Answer from the drawing. Dimensions are ordinates in mm from the lowest x, y and z of the part. A direction names the side the tool comes from. Round coordinates to 2 decimals unless told otherwise and drop trailing zeros. Order: outer loops, then holes, each group sorted by start corner. A loop starts at its lowest first (then second) coordinate and runs counter-clockwise, first axis right, second up.
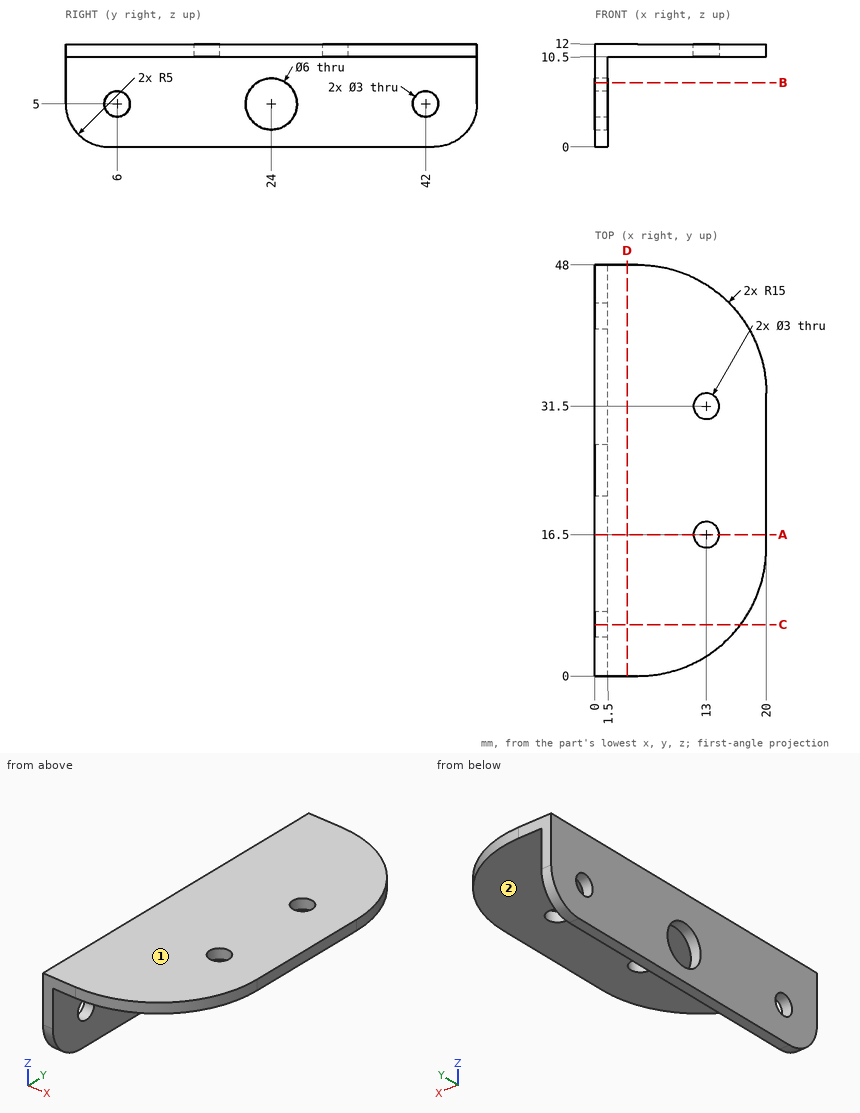
Q1. A cutting plane is placed at D-D, the plane x = 3.75. Give the vertices of the cut face in (y, z), plus the area to 3 significant figures.
Outcome:
outline: (0, 10.5) - (48, 10.5) - (48, 12) - (0, 12) - close
area: 72.0 mm2
Q2. Flat-ended cylindrical pins translate along their axes: pin 1 (4 mm diameter, centred on x = 2.5, z = 7.5, fed in from -Y); pin 2 (3 mm diameter, centred on y = 38.5, z = 8, fed in from +X); pin 3 (5.5 mm diameter, centred on x = 11.5, y = 15, fed in from -Z). Find the tip coordinate at first contact, or state that the pin passes through.
Outcome:
pin 1: stops at y = 0
pin 2: stops at x = 1.5
pin 3: stops at z = 10.5
Q3. For the marked faces 1 and 2, determine the directions among +Z, -Z, +X, -X, +Y, -Y from which every point of the face is accessible in a straight line to the end or side of a thin tool.
Outcome:
face 1: +Z, +X, -X, +Y, -Y
face 2: -Z, +X, +Y, -Y
Q4. Straight lines are drawn through the part: probe 1 along Y at (x, z) = (0.65, 5); probe 2 along Y at (x, z) = (13, 10.95); probe 3 along Z at (x, y) = (0.4, 42). For each, find the intervals that lie inside material, in ascending order.
Outcome:
probe 1: y = 0 to 4.5, 7.5 to 21, 27 to 40.5, 43.5 to 48
probe 2: y = 2.31 to 15, 18 to 30, 33 to 45.69
probe 3: z = 0 to 3.5, 6.5 to 12
Q5. A cutting plane is placed at B-B, the plane z = 7.5. Give the vertices of the cut face in (x, y).
Outcome:
outline: (0, 0) - (1.5, 0) - (1.5, 22.34) - (0, 22.34) - close; (0, 25.66) - (1.5, 25.66) - (1.5, 48) - (0, 48) - close
Q6. A cutting plane is placed at C-C, the plane y = 6. Give the vertices of the cut face in (x, z), plus the area to 4 significant figures.
Outcome:
outline: (0, 0) - (1.5, 0) - (1.5, 3.5) - (0, 3.5) - close; (0, 6.5) - (1.5, 6.5) - (1.5, 10.5) - (17, 10.5) - (17, 12) - (0, 12) - close
area: 36.75 mm2
Q7. A cutting plane is placed at A-A, the plane y = 16.5. Give the vertices of the cut face in (x, z), plus the area to 4 significant figures.
Outcome:
outline: (0, 0) - (1.5, 0) - (1.5, 10.5) - (11.5, 10.5) - (11.5, 12) - (0, 12) - close; (14.5, 10.5) - (20, 10.5) - (20, 12) - (14.5, 12) - close
area: 41.25 mm2
